Verification items for this drawing (mm, ordinates from the low corner). A direction names the side the tool comes from. Coordinates: 2 decimals unless noted, no trailing zeros. Order: outer loops, then holes, each group sorted by start corner. A loop starts at its lowest first (then second) coordinate and runs counter-clockwise, first axis right, second up. Notation, with made-up numbers: M 52,34 L 69,34 A20 ccw 69,40 Z; hole C 31,-29.5 d10. An arc over 180 degrees is marked long. Write item = value, one per line.
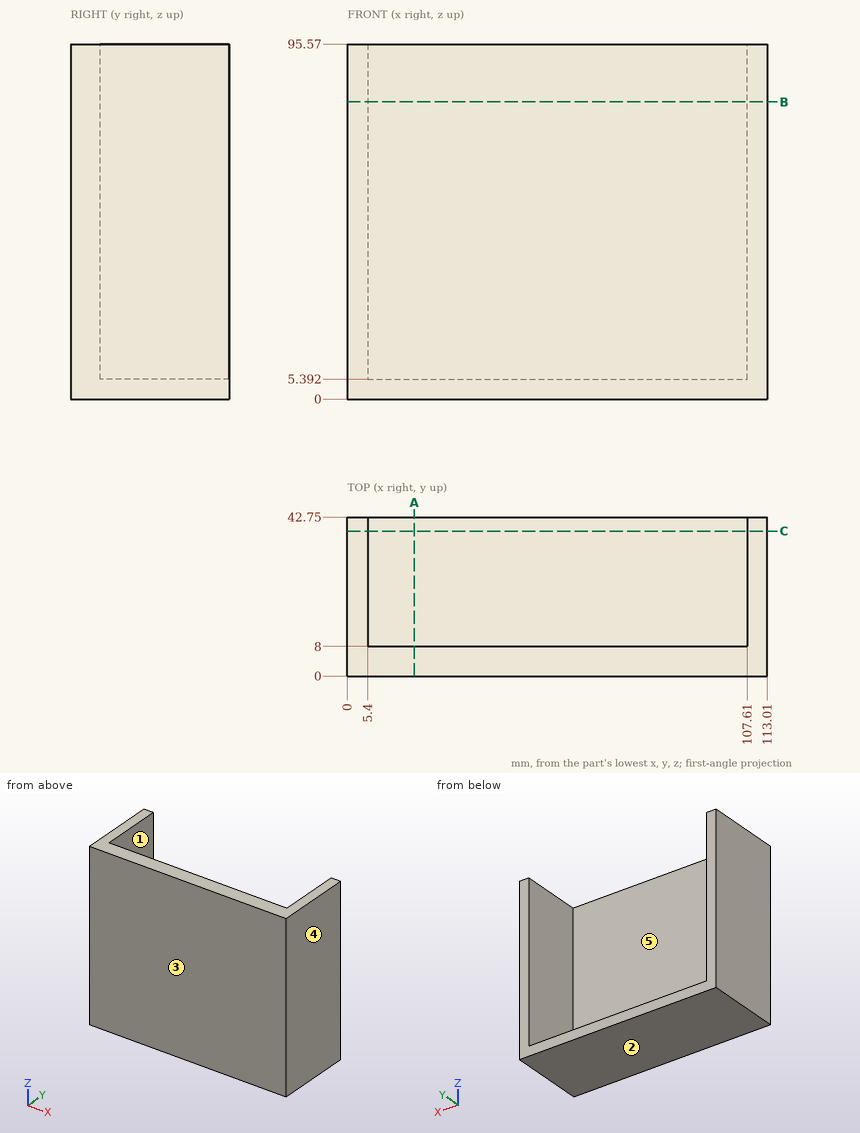
Item 1: Sectioned sample at A-A, the plane x = 18. Enter the section's corners in (y, z), then the cut area to 3 significant figures.
Report:
outline = M 0,0 L 42.75,0 L 42.75,5.39 L 8,5.39 L 8,95.57 L 0,95.57 Z
area = 952 mm^2
Item 2: Release check for a two-part mould opening along X. For the marked faces 3, 4 and 5 record: pulls with the +X half, pulls with the -X half, needs draft (parallel to the pull), parting line crosses it, or undercut.
Report:
face_3 = needs draft
face_4 = pulls with the +X half
face_5 = undercut
Item 3: Sectioned sample at B-B, the plane z = 80. Enter the section's corners in (x, y).
Report:
outline = M 0,0 L 113.01,0 L 113.01,42.75 L 107.61,42.75 L 107.61,8 L 5.4,8 L 5.4,42.75 L 0,42.75 Z
Item 4: Scan lines: L1, parallel to X at y = 32, z = 12; L2, parallel to Y at x = 33.5, z = 48.5; L3, parallel to Z at x = 46, y = 25. Record each from-to range of solid material in increasing order. Write a range as from..to.
Report:
L1 = 0..5.4, 107.61..113.01
L2 = 0..8
L3 = 0..5.39
Item 5: Gauge pin test, flat ends, axial feed: pin 1 (10 mm diameter, centred on x = 84.5, z = 79, fed in from +Y); pin 2 (12 mm diameter, centred on x = 92.5, y = 23.5, fed in from +Z). Record the tip position at first contact, or that the pin passes through.
Report:
pin_1 = 8
pin_2 = 5.39
Item 6: Sectioned sample at C-C, the plane y = 39. Enter the section's corners in (x, z).
Report:
outline = M 0,0 L 113.01,0 L 113.01,95.57 L 107.61,95.57 L 107.61,5.39 L 5.4,5.39 L 5.4,95.57 L 0,95.57 Z
Item 7: Tool access check on the marked faces 1 and 2. Record the directions out of +Z, -Z, +X, -X, +Y, -Y that give a thin tool (end or side, any length) a straight path to the whole face; none if there is none.
Report:
face_1 = +Z, +Y
face_2 = -Z, +X, -X, +Y, -Y
